Work out the finished part from the listing and answer in its coordinate system (mm). A direction names the side the tool comes from. Coordinates: 2 decimals unless noted, no trailing zeros. Order: outer loops, then holes, each group sorted by start corner. A loop starts at its lowest first (then second) coordinate and runs counter-clockwise, first axis right, second up. Notation, with made-up numbers: (-13.5, 59) - (1.5, 59) arc R34 cw to (1.5, 91) - close; hole circle Ø5 at (43, -37). An arc over 180 degrees is marked (long way). Answer as a JSON object with one key per item and string values. Group by question number.
1) Find the intervals of material crossed by line 1 along Y through (x, z) = (0, 7.5) (3 decimals); line 2 along X through (y, z) = (1, 9); line 3 along X through (y, z) = (3, 4.5), in increasing order.
2) Section B-B (z = 4) is taken. Give the vertices of the cut face in (x, y) (3 decimals), plus the area to 3 significant figures.
3) Each of these flat-tipped pins is pushed along its axis until it touches: P1, Ø3, axis at x = -10, y = -11.5, coming from the -Z side; P2, Ø1.5, axis at x = 7.5, z = 7, coming from the -Y side; P3, Ø5, axis at y = 5, z = 7, coming from the -X side; P4, Ø1, axis at y = -10.5, z = 5.5, coming from the +X side. Where does it stop, or does it pass through?
4) A tool of negligible diameter and unlimited length cuts with its end or side. For faces 4 (the face through (-1, 5, 2.54)), 5 (the face through (1, 4, 12.7)), from which of +Z, -Z, +X, -X, +Y, -Y can it reach the whole face along a straight path? Write none if from no direction.
5) The mould has two halves that part along X. Classify faces 1 (the face through (-3.555, 27.073, 6.297)), 2 (the face through (-0.83, -3.72, 6.26)), 3 (the face through (5, 0, 0)): released by +X, released by -X, zero draft, split by the parting line, or undercut.
6) Section A-A (y = 0) is taken. Give the vertices of the cut face in (x, z) (3 decimals), plus the area to 3 significant figures.
from build123d import *

# Parameters (mm, degrees)
SKETCH1_R           = 27.305
SKETCH1_R_2         = 3.81
BOSS_EXTRUDE1_DEPTH = 12.7
SKETCH2_R           = 6.089197758
SKETCH2_R_2         = 4.626410668
CUT_EXTRUDE1_DEPTH  = 10.16
FILLET2_R           = 2.54
FILLET3_R           = 2.54


with BuildPart() as part:
    # Sketch1 → Boss-Extrude1 (new body)
    with BuildSketch(Plane.XY):
        Circle(SKETCH1_R)
        Circle(SKETCH1_R_2, mode=Mode.SUBTRACT)
    extrude(amount=BOSS_EXTRUDE1_DEPTH)

    # Sketch2 → Cut-Extrude1 (cut)
    with BuildSketch(Plane.XY.offset(12.7)):
        Circle(SKETCH2_R)
        Circle(SKETCH2_R_2, mode=Mode.SUBTRACT)
    extrude(amount=-CUT_EXTRUDE1_DEPTH, mode=Mode.SUBTRACT)

    # Fillet2
    fillet2_edges = [part.edges().sort_by_distance(p)[0] for p in [
        (-6.089197758, 0, 12.7),
        (-27.305, 0, 12.7),
    ]]
    fillet(fillet2_edges, radius=FILLET2_R)

    # Fillet3
    fillet3_edges = [part.edges().sort_by_distance(p)[0] for p in [
        (-27.305, 0, 0),
    ]]
    fillet(fillet3_edges, radius=FILLET3_R)


solid = part.part
Report:
{
 "1": {"line 1": "y = -27.305 to -6.089, -4.626 to -3.81, 3.81 to 4.626, 6.089 to 27.305", "line 2": "x = -27.29 to -6.01, -4.52 to -3.68, 3.68 to 4.52, 6.01 to 27.29", "line 3": "x = -27.14 to -5.3, -3.52 to -2.35, 2.35 to 3.52, 5.3 to 27.14"},
 "2": {"outline": "circle Ø54.61 at (0, 0); circle Ø9.253 at (0, 0); hole circle Ø12.178 at (0, 0); hole circle Ø7.62 at (0, 0)", "area": "2,250 mm²"},
 "3": {"P1": "stops at z = 0", "P2": "stops at y = -26.46", "P3": "stops at x = -27.19", "P4": "stops at x = 25.41"},
 "4": {"face 4": "+Z", "face 5": "+Z, +X, -X, +Y, -Y"},
 "5": {"face 1": "split by the parting line", "face 2": "undercut", "face 3": "zero draft"},
 "6": {"outline": "(-27.305, 2.54) arc R2.54 ccw to (-24.765, 0) - (-3.81, 0) - (-3.81, 12.7) - (-4.626, 12.7) - (-4.626, 2.54) - (-6.089, 2.54) - (-6.089, 10.16) arc R2.54 ccw to (-8.629, 12.7) - (-24.765, 12.7) arc R2.54 ccw to (-27.305, 10.16) - close; (3.81, 0) - (24.765, 0) arc R2.54 ccw to (27.305, 2.54) - (27.305, 10.16) arc R2.54 ccw to (24.765, 12.7) - (8.629, 12.7) arc R2.54 ccw to (6.089, 10.16) - (6.089, 2.54) - (4.626, 2.54) - (4.626, 12.7) - (3.81, 12.7) - close", "area": "559 mm²"}
}
